The model under review builds one solid part; all positions refer to its coordinate system, in mm. Face numbers are marked on the shaded views. A direction names the side the tool comes from. Coordinates: 2 decimals unless noted, no trailing zeros. Loops run counter-clockwise (first coordinate to the right, second up) from the corner with the lowest first, then second, coordinate; pieces in that order, holes last. Notation, with made-up numbers: M 86.25,46 L 144.25,46 A27 ccw 144.25,73 Z; hole C 64.5,86 d6. An arc over 180 degrees is marked long. Return JSON: item names as keys, results as strings.
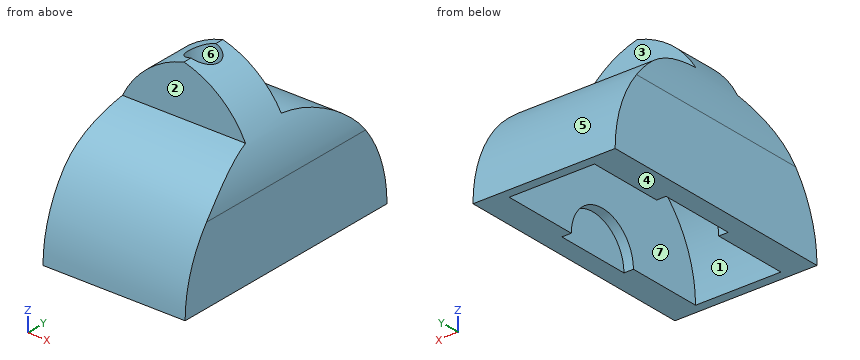
```python
from build123d import *

# Parameters (mm, degrees)
SKETCH1_W           = 15
SKETCH1_H           = 26
BOSS_EXTRUDE1_DEPTH = 18
SKETCH2_R           = 4
CUT_EXTRUDE1_DEPTH  = 11
SKETCH3_R           = 12
CUT_EXTRUDE2_DEPTH  = 9
CUT_EXTRUDE3_START  = -15
SKETCH4_W           = 45.765044891
SKETCH4_H           = 35.646606974
CUT_EXTRUDE3_DEPTH  = 15
FILLET1_R           = 10
SKETCH5_R           = 1.6
CUT_EXTRUDE4_DEPTH  = 5


with BuildPart() as part:
    # Sketch1 → Boss-Extrude1 (new body)
    with BuildSketch(Plane.XY):
        with Locations((7.5, 13)):
            Rectangle(SKETCH1_W, SKETCH1_H)
    extrude(amount=BOSS_EXTRUDE1_DEPTH)

    # Sketch2 → Cut-Extrude1 (cut)
    with BuildSketch(Plane(origin=(13, 0, 0), x_dir=(0, 0, -1), z_dir=(1, 0, 0))):
        with Locations((0, 13)):
            Circle(SKETCH2_R)
    extrude(amount=-CUT_EXTRUDE1_DEPTH, mode=Mode.SUBTRACT)

    # Sketch3 → Cut-Extrude2 (cut)
    with BuildSketch(Plane(origin=(12, 0, 0), x_dir=(0, 0, -1), z_dir=(1, 0, 0))):
        with Locations((0, 13)):
            Circle(SKETCH3_R)
    extrude(amount=-CUT_EXTRUDE2_DEPTH, mode=Mode.SUBTRACT)

    # Sketch4 → Cut-Extrude3 (cut)
    with BuildSketch(Plane(origin=(15, 0, 0), x_dir=(0, 0, -1), z_dir=(1, 0, 0)).offset(CUT_EXTRUDE3_START)):
        with Locations((-7.490754188, 14.288489829)):
            Rectangle(SKETCH4_W, SKETCH4_H)
        with BuildLine():
            Line((-20.423780573, 14), (-12.961481397, 14))
            ThreePointArc((-12.961481397, 14), (12.909776733, 14.528942348), (-12.369316877, 9))
            Line((-12.369316877, 9), (-20.423780573, 9))
            Line((-20.423780573, 9), (-20.423780573, 14))
        make_face(mode=Mode.SUBTRACT)
    extrude(amount=CUT_EXTRUDE3_DEPTH, mode=Mode.SUBTRACT)

    # Fillet1
    # the kernel refuses this fillet: 10 mm, written as the material it takes off along each edge
    with BuildSketch(Plane(origin=(15, -16, 18), x_dir=(0, 0, -1), z_dir=(0, 1, 0)), Plane(origin=(0, 39, 18), x_dir=(0, 0, -1), z_dir=(0, -1, 0))) as fillet1_piece_1:
        with BuildLine():
            CenterArc((FILLET1_R, FILLET1_R), FILLET1_R, 180, 90)
            Line((0, FILLET1_R), (0, 0))
            Line((0, 0), (FILLET1_R, 0))
        make_face()
    extrude(amount=55, mode=Mode.SUBTRACT)

    # Sketch5 → Cut-Extrude4 (cut)
    with BuildSketch(Plane.XY.offset(18)):
        with Locations((7.5, 11.5)):
            Circle(SKETCH5_R)
    extrude(amount=-CUT_EXTRUDE4_DEPTH, mode=Mode.SUBTRACT)


solid = part.part
```
1. The part is to be moulded in two halves that separate along Y. For the marked faces 4, 5, 6 and 7, say which applies: released by +Y, released by -Y, zero draft, split by the parting line, or undercut.
Check values:
{"face 4": "zero draft", "face 5": "released by +Y", "face 6": "undercut", "face 7": "undercut"}
2. Add section A-A on y = 12. Give the boundary of the cut face in (x, z), plus the area to 3 significant figures.
Check values:
{"outline": "M 0,0 L 2,0 L 2,3.87 L 3,3.87 L 3,11.96 L 12,11.96 L 12,3.87 L 13,3.87 L 13,0 L 15,0 L 15,8 A10 ccw 9.02,17.16 L 9.02,13 L 5.98,13 L 5.98,17.16 A10 ccw 0,8 Z", "area": "98.7 mm²"}
3. To check wall thickness, follow line 1 (Y direction, x = 7.5, z = 16.7); line 2 (X direction, y = 19, z = 1.75); line 3 (Y direction, x = 5, z = 6.75). State the ranges of each line that lie inside material, in increasing order.
Check values:
{"line 1": "9 to 9.9, 13.1 to 14", "line 2": "0 to 3, 12 to 15", "line 3": "1.89 to 3.08, 22.92 to 24.11"}
4. Add section C-C on z = 9. Give the boundary of the cut face in (x, y).
Check values:
{"outline": "M 0.05,3.62 L 14.95,3.62 L 14.95,22.38 L 0.05,22.38 Z; hole M 3,5.06 L 12,5.06 L 12,20.94 L 3,20.94 Z"}
5. Machinability: for the marked faces 1, 2 and 3, which of the approach directions +Z, -Z, +X, -X, +Y, -Y give a long, thin tool a straight path to every point of the face, cutting with its end or side? Answer none if there is none.
Check values:
{"face 1": "-Z", "face 2": "+Z, +X, -X, -Y", "face 3": "+Z, +X, -X, +Y"}
6. Add section D-D on y = 22.25. Give the boundary of the cut face in (x, z), plus the area to 3 significant figures.
Check values:
{"outline": "M 0,0 L 3,0 L 3,7.64 L 12,7.64 L 12,0 L 15,0 L 15,8 A10 ccw 14.94,9.13 L 0.06,9.13 A10 ccw 0,8 Z", "area": "68.2 mm²"}
7. Add section B-B on x = 3.75. Give the boundary of the cut face in (y, z), plus the area to 3 significant figures.
Check values:
{"outline": "M 0,0 L 1,0 A12 cw 25,0 L 26,0 A13 ccw 14,12.96 L 14,15.81 L 9,15.81 L 9,12.37 A13 ccw Z", "area": "54.1 mm²"}
8. Insertion check: pin 1 Ø4 at (y, z) = (5.5, 10.5) entering from +X; pin 2 Ø2.5 at (x, z) = (8.5, 16.5) entering from -Y; pin 3 Ø3 at (x, y) = (7.5, 11.5) entering from -Z. Each pin has a flat end and moves straight along its axis. Give the tip position at first contact, or say it passes through.
Check values:
{"pin 1": "x = 14.99", "pin 2": "y = 9", "pin 3": "z = 11.62"}
